```python
from build123d import *

# Parameters (mm, degrees)
SKETCH1_W           = 50
SKETCH1_H           = 187.5
BOSS_EXTRUDE1_DEPTH = 5
SKETCH2_R           = 4.9
BOSS_EXTRUDE2_DEPTH = 10
SKETCH3_W           = 25
SKETCH3_H           = 100
CUT_EXTRUDE1_DEPTH  = 10


with BuildPart() as part:
    # Sketch1 → Boss-Extrude1 (new body)
    with BuildSketch(Plane.XY):
        with Locations((25, 93.75)):
            Rectangle(SKETCH1_W, SKETCH1_H)
    extrude(amount=BOSS_EXTRUDE1_DEPTH)

    # Sketch2 → Boss-Extrude2 (add)
    with BuildSketch(Plane.XY.offset(5)):
        with Locations(Location((15, 10, 0), (0, 0, 180))):
            Circle(SKETCH2_R)
        with Locations(Location((35, 170, 0), (0, 0, 180))):
            Circle(SKETCH2_R)
    extrude(amount=BOSS_EXTRUDE2_DEPTH)

    # Sketch3 → Cut-Extrude1 (cut)
    with BuildSketch(Plane.XY.offset(5)):
        with Locations((12.5, 137.5)):
            Rectangle(SKETCH3_W, SKETCH3_H)
    extrude(amount=-CUT_EXTRUDE1_DEPTH, mode=Mode.SUBTRACT)


solid = part.part
```
The listing builds one solid part. Answer for the finished solid, in the listing's coordinates (mm). A direction names the side the tool comes from. Coordinates: 2 decimals unless noted, no trailing zeros. Write each loop counter-clockwise with the first axis right and the second up, starting at its lowest first coordinate (ties: lowest second). Pieces come first, ordered by that corner, then holes. Notation, with made-up numbers: M -24.5,45 L 27.5,45 A10 cw 27.5,53 Z; hole C 50,39.5 d6. An arc over 180 degrees is marked long. Use a Markdown table: item, result. Add a question column.
1. Which of the six approach directions +Z, -Z, +X, -X, +Y, -Y give full straight-line access (tool end or side, diameter ignored) to faces 1 (the flat face through (12, 87.5, 3)), 2 (the cylindrical face through (36.062, 174.783, 9.93)), 3 (the flat face through (15, 10, 15))?
2. Section C-C (z = 6.75) is taken. Give the vertices of the cut face in (x, y).
3. Section A-A (x = 15) is taken. Give the vertices of the cut face in (y, z), plus the area to 4 significant figures.
4. Given P1, Ø1.5, axis at x = 20, z = 2, coming from the +Y side; P2, Ø1.5, axis at x = 12.5, z = 9, coming from the +Y side; P3, Ø1.5, axis at y = 140, z = 2.5, coming from the -X side, each flat-ended and moving along its own axis, determine where each tip first touches the part or whether it passes through.
5. Section B-B (y = 170) is taken. Give the vertices of the cut face in (x, z), plus the area to 3 significant figures.
6. Section D-D (y = 36) is taken. Give the vertices of the cut face in (x, z).
7. Straight lines are drawn through the part: line 1 along Y through (x, z) = (10, 3); line 2 along X through (y, z) = (154, 4.75); line 3 along Z through (x, y) = (42, 173.5). For each, find the intervals that lie inside material, in ascending order. Write a range as [from, to].
Data:
| question | item | result |
|---|---|---|
| 1 | face 1 | +Z, -Z, -X, +Y |
| 1 | face 2 | +Z |
| 1 | face 3 | +Z, +X, -X, +Y, -Y |
| 2 | outline | C 15,10 d9.8; C 35,170 d9.8 |
| 3 | outline | M 0,0 L 87.5,0 L 87.5,5 L 14.9,5 L 14.9,15 L 5.1,15 L 5.1,5 L 0,5 Z |
| 3 | area | 535.5 mm2 |
| 4 | P1 | stops at y = 87.5 |
| 4 | P2 | stops at y = 14.58 |
| 4 | P3 | stops at x = 25 |
| 5 | outline | M 25,0 L 50,0 L 50,5 L 39.9,5 L 39.9,15 L 30.1,15 L 30.1,5 L 25,5 Z |
| 5 | area | 223 mm2 |
| 6 | outline | M 0,0 L 50,0 L 50,5 L 0,5 Z |
| 7 | line 1 | y = [0, 87.5] |
| 7 | line 2 | x = [25, 50] |
| 7 | line 3 | z = [0, 5] |
